from build123d import *

# Parameters (mm, degrees)
SKETCH1_W                  = 12.7
SKETCH1_H                  = 12.7
CUT_EXTRUDE1_DEPTH         = 6.35
CUT_EXTRUDE2_DEPTH         = 6.35
CUT_EXTRUDE3_DEPTH         = 6.35
CUT_EXTRUDE4_DEPTH         = 6.35
CUT_EXTRUDE5_DEPTH         = 6.35
CUT_EXTRUDE6_DEPTH         = 6.35
CUT_EXTRUDE7_DEPTH         = 6.35
CUT_EXTRUDE8_DEPTH         = 6.35
M3_CLEARANCE_HOLE1_D       = 3.556
M3_CLEARANCE_HOLE1_DEPTH   = 6.35
M2_5_CLEARANCE_HOLE1_D     = 2.7051
M2_5_CLEARANCE_HOLE1_DEPTH = 6.35
FILLET1_R                  = 0.8636


with BuildPart() as part:
    # Sketch1 → Revolve1 (revolve)
    with BuildSketch(Plane.XY):
        with Locations((6.35, 6.35)):
            Rectangle(SKETCH1_W, SKETCH1_H)
    revolve(axis=Axis((0, 12.7, 0), (0, -1, 0)))

    # Sketch2 → Cut-Extrude1 (cut)
    with BuildSketch(Plane(origin=(0, 12.7, 0), x_dir=(-1, 0, 0), z_dir=(0, 1, 0))):
        with BuildLine():
            Line((-5.719139865, -11.339375609), (-4.182577123, -8.292822721))
            ThreePointArc((-4.182577123, -8.292822721), (-4.751006452, -4.751006452), (-8.292822721, -4.182577123))
            Line((-8.292822721, -4.182577123), (-11.339375609, -5.719139865))
            ThreePointArc((-11.339375609, -5.719139865), (-8.980256121, -8.980256121), (-5.719139865, -11.339375609))
        make_face()
    extrude(amount=-CUT_EXTRUDE1_DEPTH, mode=Mode.SUBTRACT)

    # Sketch3 → Cut-Extrude2 (cut)
    with BuildSketch(Plane(origin=(0, 12.7, 0), x_dir=(-1, 0, 0), z_dir=(0, 1, 0))):
        with BuildLine():
            Line((-11.339375609, 5.719139865), (-8.292822721, 4.182577123))
            ThreePointArc((-8.292822721, 4.182577123), (-4.751006452, 4.751006452), (-4.182577123, 8.292822721))
            Line((-4.182577123, 8.292822721), (-5.719139865, 11.339375609))
            ThreePointArc((-5.719139865, 11.339375609), (-8.980256121, 8.980256121), (-11.339375609, 5.719139865))
        make_face()
    extrude(amount=-CUT_EXTRUDE2_DEPTH, mode=Mode.SUBTRACT)

    # Sketch4 → Cut-Extrude3 (cut)
    with BuildSketch(Plane.XZ):
        with BuildLine():
            Line((12.062191969, 3.974106807), (8.821439828, 2.906382535))
            ThreePointArc((8.821439828, 2.906382535), (6.718937759, 0), (8.821439828, -2.906382535))
            Line((8.821439828, -2.906382535), (12.062191969, -3.974106807))
            ThreePointArc((12.062191969, -3.974106807), (12.7, 0), (12.062191969, 3.974106807))
        make_face()
    extrude(amount=-CUT_EXTRUDE3_DEPTH, mode=Mode.SUBTRACT)

    # Sketch5 → Cut-Extrude4 (cut)
    with BuildSketch(Plane(origin=(0, 12.7, 0), x_dir=(-1, 0, 0), z_dir=(0, 1, 0))):
        with BuildLine():
            Line((5.719139865, 11.339375609), (4.182577123, 8.292822721))
            ThreePointArc((4.182577123, 8.292822721), (4.751006452, 4.751006452), (8.292822721, 4.182577123))
            Line((8.292822721, 4.182577123), (11.339375609, 5.719139865))
            ThreePointArc((11.339375609, 5.719139865), (8.980256121, 8.980256121), (5.719139865, 11.339375609))
        make_face()
    extrude(amount=-CUT_EXTRUDE4_DEPTH, mode=Mode.SUBTRACT)

    # Sketch6 → Cut-Extrude5 (cut)
    with BuildSketch(Plane(origin=(0, 12.7, 0), x_dir=(-1, 0, 0), z_dir=(0, 1, 0))):
        with BuildLine():
            Line((11.339375609, -5.719139865), (8.292822721, -4.182577123))
            ThreePointArc((8.292822721, -4.182577123), (4.751006452, -4.751006452), (4.182577123, -8.292822721))
            Line((4.182577123, -8.292822721), (5.719139865, -11.339375609))
            ThreePointArc((5.719139865, -11.339375609), (8.980256121, -8.980256121), (11.339375609, -5.719139865))
        make_face()
    extrude(amount=-CUT_EXTRUDE5_DEPTH, mode=Mode.SUBTRACT)

    # Sketch7 → Cut-Extrude6 (cut)
    with BuildSketch(Plane.XZ):
        with BuildLine():
            Line((3.974106807, -12.062191969), (2.906382535, -8.821439828))
            ThreePointArc((2.906382535, -8.821439828), (0, -6.718937759), (-2.906382535, -8.821439828))
            Line((-2.906382535, -8.821439828), (-3.974106807, -12.062191969))
            ThreePointArc((-3.974106807, -12.062191969), (0, -12.7), (3.974106807, -12.062191969))
        make_face()
    extrude(amount=-CUT_EXTRUDE6_DEPTH, mode=Mode.SUBTRACT)

    # Sketch8 → Cut-Extrude7 (cut)
    with BuildSketch(Plane.XZ):
        with BuildLine():
            Line((-12.062191969, -3.974106807), (-8.821439828, -2.906382535))
            ThreePointArc((-8.821439828, -2.906382535), (-6.718937759, 0), (-8.821439828, 2.906382535))
            Line((-8.821439828, 2.906382535), (-12.062191969, 3.974106807))
            ThreePointArc((-12.062191969, 3.974106807), (-12.7, 0), (-12.062191969, -3.974106807))
        make_face()
    extrude(amount=-CUT_EXTRUDE7_DEPTH, mode=Mode.SUBTRACT)

    # Sketch9 → Cut-Extrude8 (cut)
    with BuildSketch(Plane.XZ):
        with BuildLine():
            Line((-3.974106807, 12.062191969), (-2.906382535, 8.821439828))
            ThreePointArc((-2.906382535, 8.821439828), (0, 6.718937759), (2.906382535, 8.821439828))
            Line((2.906382535, 8.821439828), (3.974106807, 12.062191969))
            ThreePointArc((3.974106807, 12.062191969), (0, 12.7), (-3.974106807, 12.062191969))
        make_face()
    extrude(amount=-CUT_EXTRUDE8_DEPTH, mode=Mode.SUBTRACT)

    # Sketch10 → Cut-Revolve1 (revolve, cut)
    with BuildSketch(Plane(origin=(0, 0, 0), x_dir=(-1, 0, 0), z_dir=(0, 0, -1))):
        Polygon((-6.35, 0), (0, 0), (0, 12.7), (-6.35, 12.7), (-6.35, 7.9375), (-4.7625, 7.9375), (-4.7625, 4.7625), (-6.35, 4.7625), align=None)
    revolve(axis=Axis((0, 0, 0), (0, 1, 0)), mode=Mode.SUBTRACT)

    # M3 Clearance Hole1
    with Locations(Plane(origin=(0, 6.35, 0), x_dir=(1, 0, 0), z_dir=(0, 1, 0))):
        with Locations((6.914797213, 6.914797213), (-6.914797213, 6.914797213), (-6.914797213, -6.914797213), (6.914797213, -6.914797213)):
            Hole(M3_CLEARANCE_HOLE1_D / 2, depth=M3_CLEARANCE_HOLE1_DEPTH)

    # M2.5 Clearance Hole1
    with Locations(Plane(origin=(0, 6.35, 0), x_dir=(-1, 0, 0), z_dir=(0, -1, 0))):
        with Locations((-9.779, 0), (0, 9.779), (9.779, 0), (0, -9.779)):
            Hole(M2_5_CLEARANCE_HOLE1_D / 2, depth=M2_5_CLEARANCE_HOLE1_DEPTH)

    # Fillet1
    fillet1_edges = [part.edges().sort_by_distance(p)[0] for p in [
        (-3.974106807, 3.175, 12.062191969),
        (3.974106807, 3.175, 12.062191969),
        (5.719139865, 9.525, -11.339375609),
        (11.339375609, 9.525, -5.719139865),
        (11.339375609, 9.525, 5.719139865),
        (5.719139865, 9.525, 11.339375609),
        (12.062191969, 3.175, 3.974106807),
        (12.062191969, 3.175, -3.974106807),
        (-5.719139865, 9.525, 11.339375609),
        (-11.339375609, 9.525, 5.719139865),
        (-11.339375609, 9.525, -5.719139865),
        (-5.719139865, 9.525, -11.339375609),
        (3.974106807, 3.175, -12.062191969),
        (-3.974106807, 3.175, -12.062191969),
        (-12.062191969, 3.175, -3.974106807),
        (-12.062191969, 3.175, 3.974106807),
    ]]
    fillet(fillet1_edges, radius=FILLET1_R)


solid = part.part
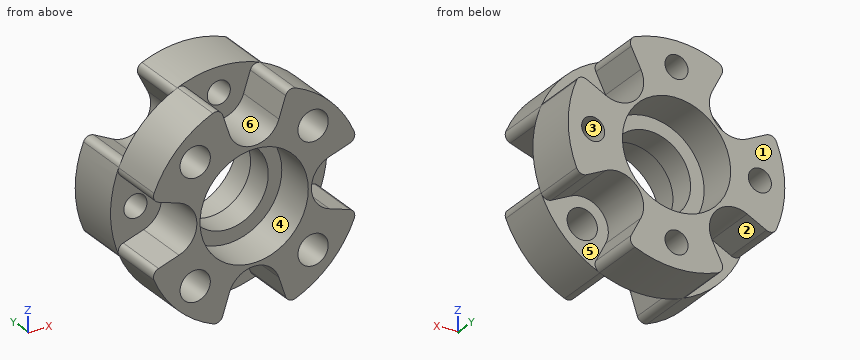
Source: CAD feature listing. Evaluate the final solid. Frame: model axes, mm. Face numbers are marked on the shaded views. A direction names the side the tool comes from. Round coordinates to 2 decimals unless told otherwise and drop trailing zeros. Write each loop counter-clockwise with the first axis right and the second up, starting at its lowest first coordinate (ties: lowest second). Pieces come first, ordered by that corner, then holes. Notation, with made-up numbers: (58, 79) - (101, 79) arc R25 ccw to (101, 103) - close; hole circle Ø7 at (-6, 87.5). An arc over 180 degrees is marked (long way). Use CSV: the item, a comma, the result in double quotes. Start each with the question number.
(1) Set-up query: the marked faces 4, 5 and 6. Return all of +Z, -Z, +X, -X, +Y, -Y with unobstructed straight access to the full face (end or side cutting, diameter ignored); none if empty.
(2) Cut plane D-D, the plane z = -7.5. Return loops of the section in (x, y), and give its area (3 significant figures).
(3) Cut plane C-C, the plane x = 6. Return loops of the section in (y, z).
(4) Material intervals for probe 1 along Z at (x, y) = (0, 8.9); probe 2 along Z at (x, y) = (0, 7.05); probe 3 along X at (y, z) = (12.25, -4.75), sorted ascending. Write a range as [from, to].
(5) Cut plane A-A, the plane x = 0. Return loops of the section in (y, z).
(6) First-contact query: pin 1 Ø6.5 at (x, z) = (2, -1.5) entering from -Y; pin 2 Ø2 at (x, y) = (-4.5, 9) entering from -Z; pin 3 Ø4.5 at (x, z) = (6.91, -6.91) entering from +Y. Flat tips, straight axial feed; report the tip coordinate or a pass-through.
(7) Mould query, pull axis Z, two halves, no side actions, for the marked faces 1, 2 and 3. Classes: pulls with the +Z half, pulls with the -Z half, needs draft (parallel to the pull), parting line crosses it, or undercut.
(8) Cut plane B-B, the plane z = 0. Return loops of the section in (x, y).
Geometry says:
1,face 4,"-Y"
1,face 5,"+Y"
1,face 6,"+Z, -Y"
2,outline,"(-10.25, 0) - (-8.59, 0) - (-8.59, 6.35) - (-10.25, 6.35) - close; (-5.24, 0) - (-2.04, 0) - (-2.04, 6.35) - (2.04, 6.35) - (2.04, 0) - (5.24, 0) - (5.24, 6.35) - (3.91, 6.35) - (3.91, 12.7) - (-3.91, 12.7) - (-3.91, 6.35) - (-5.24, 6.35) - close; (8.59, 0) - (10.25, 0) - (10.25, 6.35) - (8.59, 6.35) - close"
2,area,"111 mm²"
3,outline,"(0, -11.19) - (6.35, -11.19) - (6.35, -8.44) - (0, -8.44) - close; (0, -5.39) - (6.35, -5.39) - (6.35, -3.99) - (12.7, -3.99) - (12.7, -2.08) - (7.94, -2.08) - (7.94, 2.08) - (12.7, 2.08) - (12.7, 3.99) - (6.35, 3.99) - (6.35, 5.39) - (0, 5.39) - (0, 2.08) - (4.76, 2.08) - (4.76, -2.08) - (0, -2.08) - close; (0, 8.44) - (6.35, 8.44) - (6.35, 11.19) - (0, 11.19) - close"
4,probe 1,"[-12.7, -11.13], [-8.43, -6.35], [6.35, 8.43], [11.13, 12.7]"
4,probe 2,"[-12.7, -11.13], [-8.43, -4.76], [4.76, 8.43], [11.13, 12.7]"
4,probe 3,"[-11.78, -9.42], [-4.75, -4.21], [4.21, 4.75], [9.42, 11.78]"
5,outline,"(0, -6.72) - (6.35, -6.72) - (6.35, -8.43) - (12.7, -8.43) - (12.7, -6.35) - (7.94, -6.35) - (7.94, -4.76) - (4.76, -4.76) - (4.76, -6.35) - (0, -6.35) - close; (0, 6.35) - (4.76, 6.35) - (4.76, 4.76) - (7.94, 4.76) - (7.94, 6.35) - (12.7, 6.35) - (12.7, 8.43) - (6.35, 8.43) - (6.35, 6.72) - (0, 6.72) - close; (6.35, -12.7) - (12.7, -12.7) - (12.7, -11.13) - (6.35, -11.13) - close; (6.35, 11.13) - (12.7, 11.13) - (12.7, 12.7) - (6.35, 12.7) - close"
6,pin 1,"y = 4.76"
6,pin 2,"z = -12.21"
6,pin 3,"y = 6.35"
7,face 1,"needs draft"
7,face 2,"pulls with the -Z half"
7,face 3,"undercut"
8,outline,"(-12.7, 6.35) - (-11.13, 6.35) - (-11.13, 12.7) - (-12.7, 12.7) - close; (-8.43, 6.35) - (-6.72, 6.35) - (-6.72, 0) - (-6.35, 0) - (-6.35, 4.76) - (-4.76, 4.76) - (-4.76, 7.94) - (-6.35, 7.94) - (-6.35, 12.7) - (-8.43, 12.7) - close; (4.76, 4.76) - (6.35, 4.76) - (6.35, 0) - (6.72, 0) - (6.72, 6.35) - (8.43, 6.35) - (8.43, 12.7) - (6.35, 12.7) - (6.35, 7.94) - (4.76, 7.94) - close; (11.13, 6.35) - (12.7, 6.35) - (12.7, 12.7) - (11.13, 12.7) - close"
